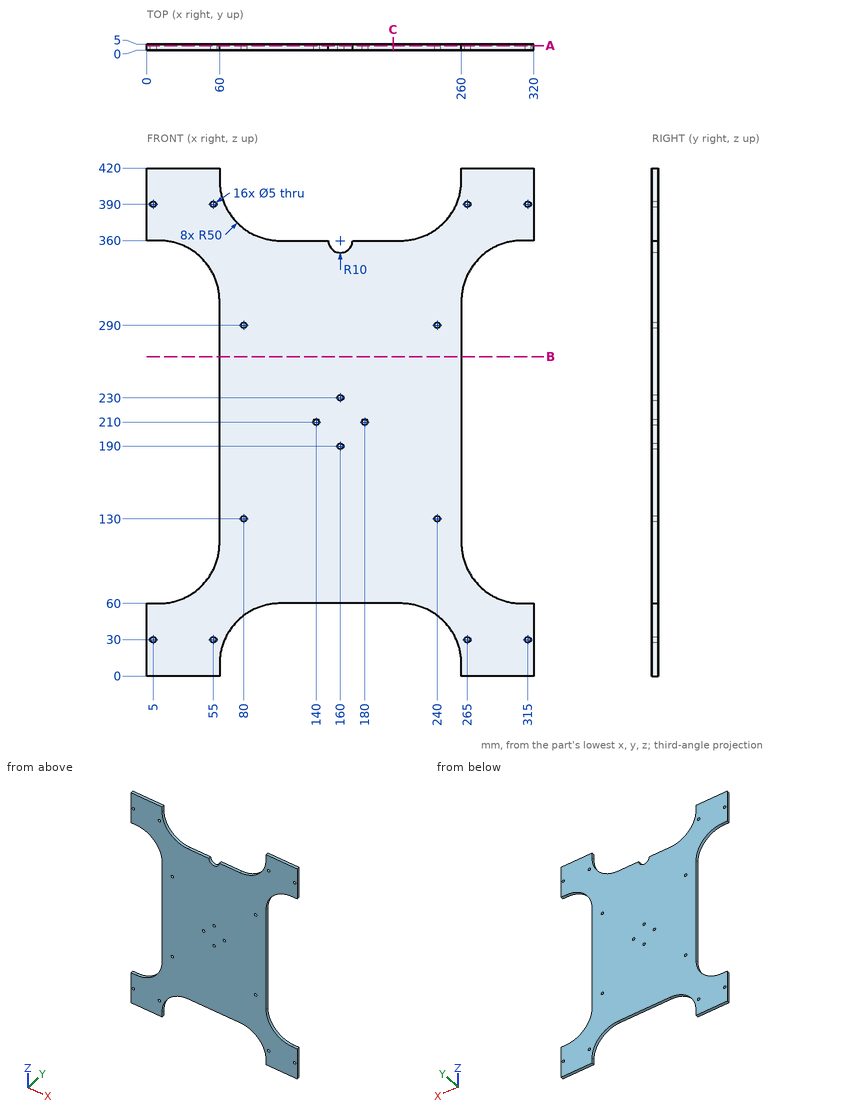
Job drawing, mm, ordinate dimensions from the low corner. One solid piece. Coordinates: 2 decimals unless noted, no trailing zeros. Order: outer loops, then holes, each group sorted by start corner. A loop starts at its lowest first (then second) coordinate and runs counter-clockwise, first axis right, second up. Notation, with made-up numbers: M 86.25,78.5 L 115.25,78.5 A21 ccw 115.25,102.5 Z; hole C 52,63.5 d5. An arc over 180 degrees is marked long. Answer as CSV lines item,"result".
(1) Band-saw the part on B-B, the plane z = 264. List the corners of the cut face in (x, y), then the cut area to 3 significant figures.
Geometry says:
outline,"M 60,0 L 260,0 L 260,5 L 60,5 Z"
area,"1,000 mm2"
(2) Band-saw the part on C-C, the plane x = 203.5. List the corners of the cut face in (y, z), then the cut area to 3 significant figures.
Geometry says:
outline,"M 0,60 L 5,60 L 5,360 L 0,360 Z"
area,"1,500 mm2"
(3) Wall check: line 1 along Z through (x, y) = (160, 3.7); line 2 along Z through (x, y) = (315, 3.3); line 3 along Z through (x, y) = (140, 1.8). Give the ranges that are in metal, low to high.
Geometry says:
line 1,"z = 60 to 187.5, 192.5 to 227.5, 232.5 to 350"
line 2,"z = 0 to 27.5, 32.5 to 60, 360 to 387.5, 392.5 to 420"
line 3,"z = 60 to 207.5, 212.5 to 360"
(4) Flat gauge pins, fed straight in: pin 1 (3 mm diameter, centred on x = 240, z = 130, fed in from +Y); pin 2 (1.5 mm diameter, centred on x = 198, y = 3, fed in from +Z); pin 3 (2 mm diameter, centred on y = 2.5, z = 249.5, fed in from +X); pin 4 (2 mm diameter, centred on x = 163.5, y = 0.5, fed in from +Z). Where does each tip first touch, or does it go through?
Geometry says:
pin 1,"passes through"
pin 2,"stops at z = 360"
pin 3,"stops at x = 260"
pin 4,"stops at z = 351.07"
(5) Band-saw the part on A-A, the plane y = 3.65. State how many separate pieces and enclosed holes the cut face has, then the cut area to 3 significant figures.
Geometry says:
separate pieces,"1"
enclosed holes,"16"
area,"78,200 mm2"
